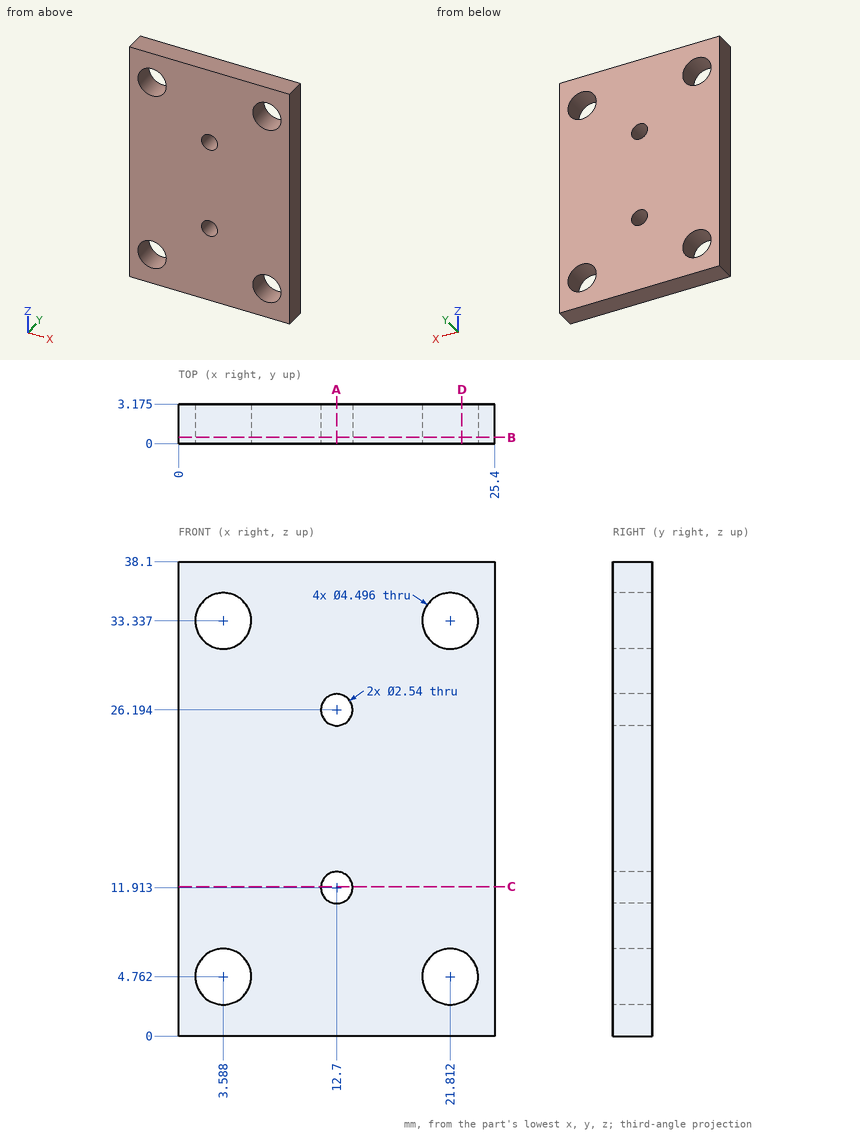
The figure shows three views and two pictorial views of one solid part (mm, origin at its lowest corner). Answer the questions. Give positions to 0.01 mm unless a question says otherwise; leave off trailing zeros. Write each loop counter-clockwise with the first axis right and the second up, starting at its lowest first coordinate (ties: lowest second). Pieces come first, ordered by that corner, then holes. Notation, with made-up numbers: (-32, 60.5) - (12, 60.5) arc R11 ccw to (12, 66.5) - close; hole circle Ø1 at (39, 20). An arc over 180 degrees is marked (long way). Return JSON: item names as keys, results as strings.
Q1. A cutting plane is placed at A-A, the plane x = 12.7. Determine the outline of the cut face in (y, z) (1 decimal), and give its area (3 significant figures).
Reply:
{"outline": "(0, 0) - (3.2, 0) - (3.2, 10.6) - (0, 10.6) - close; (0, 13.2) - (3.2, 13.2) - (3.2, 24.9) - (0, 24.9) - close; (0, 27.5) - (3.2, 27.5) - (3.2, 38.1) - (0, 38.1) - close", "area": "105 mm²"}
Q2. A cutting plane is placed at C-C, the plane z = 12. Determine the outline of the cut face in (x, y) (1 decimal).
Reply:
{"outline": "(0, 0) - (11.4, 0) - (11.4, 3.2) - (0, 3.2) - close; (14, 0) - (25.4, 0) - (25.4, 3.2) - (14, 3.2) - close"}
Q3. A cutting plane is placed at B-B, the plane y = 0.5. Determine the outline of the cut face in (x, z) (1 decimal).
Reply:
{"outline": "(0, 0) - (25.4, 0) - (25.4, 38.1) - (0, 38.1) - close; hole circle Ø4.5 at (3.6, 4.8); hole circle Ø4.5 at (3.6, 33.3); hole circle Ø2.5 at (12.7, 11.9); hole circle Ø2.5 at (12.7, 26.2); hole circle Ø4.5 at (21.8, 4.8); hole circle Ø4.5 at (21.8, 33.3)"}
Q4. Consider line 1 along Z through (x, y) = (3.5, 1.4); line 2 along Z through (x, y) = (12.7, 2.2); line 3 along X through (y, z) = (1.3, 5). Determine where each line is inside the solid, lowest interval first. Write a range as [from, to].
Reply:
{"line 1": "[0, 2.52], [7.01, 31.09], [35.58, 38.1]", "line 2": "[0, 10.64], [13.18, 24.92], [27.46, 38.1]", "line 3": "[0, 1.35], [5.82, 19.58], [24.05, 25.4]"}
Q5. A cutting plane is placed at D-D, the plane x = 22.75. Determine the outline of the cut face in (y, z) (1 decimal).
Reply:
{"outline": "(0, 0) - (3.2, 0) - (3.2, 2.7) - (0, 2.7) - close; (0, 6.8) - (3.2, 6.8) - (3.2, 31.3) - (0, 31.3) - close; (0, 35.4) - (3.2, 35.4) - (3.2, 38.1) - (0, 38.1) - close"}
Q6. Given P1, Ø2.5, axis at x = 3.59, z = 4.76, coming from the -Y side, flat-ended and moving along its own axis, determine where the tip first touches the part or whether it passes through.
Reply:
{"P1": "through"}
